from build123d import *

# Parameters (mm, degrees)
SKETCH1_R           = 11.5
SHAFT_DEPTH         = 50
BOSS_EXTRUDE2_DEPTH = 50
FILLET1_R           = 10
CIRPATTERN1_START   = -50
CIRPATTERN1_DEPTH   = 56.614378378


with BuildPart() as part:
    # Sketch1 → Shaft (new, symmetric)
    with BuildSketch(Plane.XY):
        Circle(SKETCH1_R)
    extrude(amount=SHAFT_DEPTH, both=True)

    # Sketch2 → Boss-Extrude2 (add)
    with BuildSketch(Plane.XY):
        with BuildLine():
            Line((3, 11.101801656), (3, 13.674794331))
            ThreePointArc((3, 13.674794331), (0, 14), (-3, 13.674794331))
            Line((-3, 13.674794331), (-3, 11.101801656))
            ThreePointArc((-3, 11.101801656), (0, 11.5), (3, 11.101801656))
        make_face()
    extrude(amount=-BOSS_EXTRUDE2_DEPTH)

    # Fillet1
    # the kernel refuses this fillet: 10 mm, written as the material it adds along each edge
    with BuildSketch(Plane(origin=(0, 0, 0), x_dir=(-0.9914186895468253, -0.13072483320798547, 0), z_dir=(0.13072483320798547, -0.9914186895468253, 0))) as fillet1_piece_1_section:
        with BuildLine():
            CenterArc((21.5, -6.614378278), FILLET1_R, 138.590377891, 41.409622109)
            Line((14, 0), (13.85, 0.132287566))
            ThreePointArc((13.85, 0.132287566), (12.75, 0.2), (11.5, 0.2))
            Line((11.5, 0.2), (11.3, 0))
            Line((11.3, 0), (11.3, -6.614378278))
            Line((11.3, -6.614378278), (11.5, -6.614378278))
        make_face()
    fillet1_piece_1 = revolve(axis=Axis((0, 0, 0), (0, 0, -1)), revolution_arc=195.022959301, mode=Mode.PRIVATE)
    fillet1_piece_1 = split(fillet1_piece_1, bisect_by=Plane(origin=(-3, 0, 0), z_dir=(1, 0, 0)), keep=Keep.TOP, mode=Mode.PRIVATE)
    fillet1_piece_1 = split(fillet1_piece_1, bisect_by=Plane(origin=(3, 0, 0), z_dir=(-1, 0, 0)), keep=Keep.TOP, mode=Mode.PRIVATE)
    add(fillet1_piece_1)

    # CirPattern1: read off the stored shape, not the designer's step
    # CirPattern1 outline → CirPattern1 (add)
    with BuildSketch(Plane.XY.offset(CIRPATTERN1_START)):
        with BuildLine():
            Line((11.114442262, 2.952824616), (13.342719282, 4.239320954))
            ThreePointArc((13.342719282, 4.239320954), (12.124355653, 7), (10.342719282, 9.435473377))
            Line((10.342719282, 9.435473377), (8.114442262, 8.148977039))
            ThreePointArc((8.114442262, 8.148977039), (9.959292144, 5.75), (11.114442262, 2.952824616))
        make_face()
        with BuildLine():
            ThreePointArc((-11.114442262, 2.952824616), (-9.959292144, 5.75), (-8.114442262, 8.148977039))
            Line((-8.114442262, 8.148977039), (-10.342719282, 9.435473377))
            ThreePointArc((-10.342719282, 9.435473377), (-12.124355653, 7), (-13.342719282, 4.239320954))
            Line((-13.342719282, 4.239320954), (-11.114442262, 2.952824616))
        make_face()
        with BuildLine():
            Line((13.342719282, -4.239320954), (11.114442262, -2.952824616))
            ThreePointArc((11.114442262, -2.952824616), (9.959292144, -5.75), (8.114442262, -8.148977039))
            Line((8.114442262, -8.148977039), (10.342719282, -9.435473377))
            ThreePointArc((10.342719282, -9.435473377), (12.124355653, -7), (13.342719282, -4.239320954))
        make_face()
        with BuildLine():
            ThreePointArc((-8.114442262, -8.148977039), (-9.959292144, -5.75), (-11.114442262, -2.952824616))
            Line((-11.114442262, -2.952824616), (-13.342719282, -4.239320954))
            ThreePointArc((-13.342719282, -4.239320954), (-12.124355653, -7), (-10.342719282, -9.435473377))
            Line((-10.342719282, -9.435473377), (-8.114442262, -8.148977039))
        make_face()
        with BuildLine():
            Line((3, -13.674794331), (3, -11.101801656))
            ThreePointArc((3, -11.101801656), (0, -11.5), (-3, -11.101801656))
            Line((-3, -11.101801656), (-3, -13.674794331))
            ThreePointArc((-3, -13.674794331), (0, -14), (3, -13.674794331))
        make_face()
    extrude(amount=CIRPATTERN1_DEPTH)

    # CirPattern1 2 outline → CirPattern1 2 (revolve, cut)
    with BuildSketch(Plane.XZ):
        with BuildLine():
            ThreePointArc((11.5, 6.614378278), (12.145856533, 3.078844372), (14, 0))
            Line((14, 0), (14, 6.614378378))
            Line((14, 6.614378378), (11.5, 6.614378278))
        make_face()
    revolve(axis=Axis((0, 0, 0), (0, 0, 1)), mode=Mode.SUBTRACT)


solid = part.part
Can you work these out from the model? Positions are in its coordinate system, mm. A direction names the side the tool comes from. Round coordinates to 2 decimals unless told otherwise and drop trailing zeros. Loops run counter-clockwise (first coordinate to the right, second up) from the corner with the lowest first, then second, coordinate; pieces in that order, holes last. Notation, with made-up numbers: (-11, 36.5) - (39, 36.5) arc R25 cw to (39, 59.5) - close; hole circle Ø4 at (20.5, -29). An arc over 180 degrees is marked (long way). Answer in a Markdown table with one row per item. Add a question column.
Q1. We'd pull the mould along X, two halves only. Please class faces 5 (the flat face through (12.244, -3.605, -22.089)), 6 (the flat face through (-9.24, -8.8, -22.09)), 7 (the flat face through (-12.213, -3.587, -22.089)): pulls with the +X half, pulls with the -X half, needs draft (parallel to the pull), parting line crosses it, or undercut.
Q2. I want a section at B-B on z = -10. List the corners of the cut face in (x, y) for me.
Q3. I need wall thicknesses on L1, parallel to Y at x = -0.25, z = -43.5; L2, parallel to X at y = 12.25, z = -45.5; L3, parallel to Y at x = 3.75, z = -6.5. Which ranges of each line are inside material? Lowest first, please.
Q4. Which directions (+Z, -Z, +X, -X, +Y, -Y) give clear straight access to the entire face, cutting with the end or side of a thin tool? Please do faces 1 (the flat face through (9.24, 8.8, -22.09)), 2 (the flat face through (9.21, -8.78, -22.09)), 3 (the flat face through (3, -12, -22)), 4 (the flat face through (-3, -12, -22)).
Q5. For pin 1 Ø1 at (x, z) = (8.5, 25) entering from +Y; pin 2 Ø12 at (y, z) = (9.5, -37.5) entering from +X; pin 3 Ø1.3 at (y, z) = (-12.5, -16) entering from +X, each with a flat end and sliding along its axis, tell me the tip position at first contact or that it passes through.
Q6. I want a section at D-D on x = -4.5. List the corners of the cut face in (y, z) for me.
Q7. I want a section at C-C on y = 0. List the corners of the cut face in (x, z) for me.
Q8. I want a section at A-A on x = 0. List the corners of the cut face in (y, z) for me, and give its area (3 significant figures).
A:
| question | item | result |
|---|---|---|
| 1 | face 5 | pulls with the +X half |
| 1 | face 6 | undercut |
| 1 | face 7 | pulls with the -X half |
| 2 | outline | (-13.34, -4.24) arc R14 ccw to (-10.34, -9.44) - (-8.11, -8.15) arc R11.5 ccw to (-3, -11.1) - (-3, -13.67) arc R14 ccw to (3, -13.67) - (3, -11.1) arc R11.5 ccw to (8.11, -8.15) - (10.34, -9.44) arc R14 ccw to (13.34, -4.24) - (11.11, -2.95) arc R11.5 ccw to (11.11, 2.95) - (13.34, 4.24) arc R14 ccw to (10.34, 9.44) - (8.11, 8.15) arc R11.5 ccw to (3, 11.1) - (3, 13.67) arc R14 ccw to (-3, 13.67) - (-3, 11.1) arc R11.5 ccw to (-8.11, 8.15) - (-10.34, 9.44) arc R14 ccw to (-13.34, 4.24) - (-11.11, 2.95) arc R11.5 ccw to (-11.11, -2.95) - close |
| 3 | L1 | -14 to 14 |
| 3 | L2 | -3 to 3 |
| 3 | L3 | -10.87 to 10.87 |
| 4 | face 1 | +Z, -Z, +Y |
| 4 | face 2 | +Z, -Z, -Y |
| 4 | face 3 | +Z, -Z, +X, -Y |
| 4 | face 4 | +Z, -Z, -X, -Y |
| 5 | pin 1 | y = 8.26 |
| 5 | pin 2 | x = 13.34 |
| 5 | pin 3 | x = 3 |
| 6 | outline | (-10.58, -50) - (10.58, -50) - (10.58, 50) - (-10.58, 50) - close |
| 7 | outline | (-11.5, -50) - (11.5, -50) - (11.5, 50) - (-11.5, 50) - close |
| 8 | outline | (-14, -50) - (14, -50) - (14, 0) arc R10 cw to (11.5, 6.61) - (11.5, 50) - (-11.5, 50) - (-11.5, 6.61) arc R10 cw to (-14, 0) - close |
| 8 | area | 2,560 mm^2 |
